from build123d import *

# Parameters (mm, degrees)
F0_W     = 203.2
F0_H     = 6.35
F1_DEPTH = 35.56
F3_D     = 2.2606
F3_DEPTH = 13.74775
F3_TIP   = 0.6791527577
F5_DEPTH = 6.351


with BuildPart() as f1:
    # F0 (on Top) → F1 (new body)
    with BuildSketch(Plane.XY):
        Rectangle(F0_W, F0_H)
    extrude(amount=F1_DEPTH)

    # F3
    with Locations(Plane.XY.offset(35.56)):
        with Locations((0, 0), (88.9, 0), (-88.9, 0)):
            Hole(F3_D / 2, depth=F3_DEPTH)
            with Locations((0, 0, -(F3_DEPTH + F3_TIP / 2))):  # 118° drill point
                Cone(0, F3_D / 2, F3_TIP, mode=Mode.SUBTRACT)

    # F4 (on face) → F5 (cut, through all)
    with BuildSketch(Plane(origin=(0, 3.175, 0), x_dir=(-1, 0, 0), z_dir=(0, 1, 0))):
        with BuildLine():
            Line((70.9315911112, 24.765), (49.7184088888, 24.765))
            ThreePointArc((49.7184088888, 24.765), (47.625, 17.78), (49.7184088888, 10.795))
            Line((49.7184088888, 10.795), (70.9315911112, 10.795))
            ThreePointArc((70.9315911112, 10.795), (73.025, 17.78), (70.9315911112, 24.765))
        make_face()
        with BuildLine():
            Line((-26.4815911112, 10.795), (-5.2684088888, 10.795))
            ThreePointArc((-5.2684088888, 10.795), (-3.175, 17.78), (-5.2684088888, 24.765))
            Line((-5.2684088888, 24.765), (-26.4815911112, 24.765))
            ThreePointArc((-26.4815911112, 24.765), (-28.575, 17.78), (-26.4815911112, 10.795))
        make_face()
    extrude(amount=-F5_DEPTH, mode=Mode.SUBTRACT)


solid = f1.part
Design review of the part built by this model. Coordinates are the model's own, in mm. A direction names the side the tool comes from. Coordinates: 2 decimals unless noted, no trailing zeros. Loops run counter-clockwise (first coordinate to the right, second up) from the corner with the lowest first, then second, coordinate; pieces in that order, holes last. Notation, with made-up numbers: M -11.5,2 L 39.5,2 A20 cw 39.5,31 Z; hole C 58,34 d9. An arc over 180 degrees is marked long. Answer as CSV lines item,"result".
Item 1: The part is to be moulded in two halves that separate along X. For faces 3 (the face through (101.6, 0, 18)), 4 (the face through (-1.4, 0, 35.56)), 5 (the face through (3.175, 0.044, 17.676)), say which applies: pulls with the +X half, pulls with the -X half, needs draft (parallel to the pull), parting line crosses it, or undercut.
Answer list:
face 3,"pulls with the +X half"
face 4,"needs draft"
face 5,"undercut"
Item 2: For probe 1 along X at (y, z) = (0, 25); probe 2 along Y at (x, z) = (0, 28.5) (3 decimals); probe 3 along X at (y, z) = (-1.75, 14.5), list the stretches that pass through material, from the lowest coordinate up.
Answer list:
probe 1,"-101.6 to -90.03, -87.77 to -1.13, 1.13 to 87.77, 90.03 to 101.6"
probe 2,"-3.175 to -1.13, 1.13 to 3.175"
probe 3,"-101.6 to -72.59, -48.06 to 3.61, 28.14 to 101.6"
Item 3: Machinability: for faces 1 (the face through (28.575, 0.044, 17.884)), 2 (the face through (-1, -3.175, 18)), which of the approach directions +Z, -Z, +X, -X, +Y, -Y give a long, thin tool a straight path to every point of the face, cutting with its end or side? Answer none if there is none.
Answer list:
face 1,"+Y, -Y"
face 2,"+Z, -Z, +X, -X, -Y"
Item 4: Add section A-A on x = 21. State the section outline as (y, z) points (3 decimals), plus the area to 3 significant figures.
Answer list:
outline,"M -3.175,0 L 3.175,0 L 3.175,10.795 L -3.175,10.795 Z; M -3.175,24.765 L 3.175,24.765 L 3.175,35.56 L -3.175,35.56 Z"
area,"137 mm²"
Item 5: For P1, Ø1.4, axis at x = 0, y = 0, coming from the +Z side; P2, Ø6, axis at x = 25, z = 20.5, coming from the +Y side, all flat-tipped, find the tip position at first contact; note any pin that passes through.
Answer list:
P1,"z = 21.55"
P2,"through"
Item 6: Add section B-B on z = 18. State the section outline as (x, y) points (3 decimals), plus the area to 3 significant figures.
Answer list:
outline,"M -101.6,-3.175 L -73.023,-3.175 L -73.023,3.175 L -101.6,3.175 Z; M -47.627,-3.175 L 3.177,-3.175 L 3.177,3.175 L -47.627,3.175 Z; M 28.573,-3.175 L 101.6,-3.175 L 101.6,3.175 L 28.573,3.175 Z"
area,"968 mm²"
